from build123d import *

# Parameters (mm, degrees)
PIN_DRAWING_W       = 0.636
PIN_DRAWING_H       = 0.636
BOSS_EXTRUDE1_DEPTH = 2.54


with BuildPart() as part:
    # pin_drawing → Boss-Extrude1 (new body)
    with BuildSketch(Plane.XY):
        Polygon((0, 2.146446609), (0, 0.353553391), (0.353553391, 0), (0, -0.353553391), (0, -2.146446609), (0.353553391, -2.5), (2.187446609, -2.5), (2.541, -2.146446609), (2.541, -0.353553391), (2.187446609, 0), (2.541, 0.353553391), (2.541, 2.146446609), (2.187446609, 2.5), (2.541, 2.853553391), (2.541, 4.646446609), (2.187446609, 5), (2.541, 5.353553391), (2.541, 7.146446609), (2.187446609, 7.5), (0.353553391, 7.5), (0, 7.146446609), (0, 5.353553391), (0.353553391, 5), (0, 4.646446609), (0, 2.853553391), (0.353553391, 2.5), align=None)
        with Locations((1.2705, -1.25)):
            Rectangle(PIN_DRAWING_W, PIN_DRAWING_H, mode=Mode.SUBTRACT)
        with Locations((1.2705, 1.25)):
            Rectangle(PIN_DRAWING_W, PIN_DRAWING_H, mode=Mode.SUBTRACT)
        with Locations((1.2705, 3.75)):
            Rectangle(PIN_DRAWING_W, PIN_DRAWING_H, mode=Mode.SUBTRACT)
        with Locations((1.2705, 6.25)):
            Rectangle(PIN_DRAWING_W, PIN_DRAWING_H, mode=Mode.SUBTRACT)
    extrude(amount=BOSS_EXTRUDE1_DEPTH)


solid = part.part
Source: CAD feature listing. Evaluate the final solid. Frame: model axes, mm. Round coordinates to 2 decimals unless told otherwise and drop trailing zeros. Loops run counter-clockwise (first coordinate to the right, second up) from the corner with the lowest first, then second, coordinate; pieces in that order, holes last. Notation, with made-up numbers: M 64,10 L 118,10 A26 ccw 118,29 Z; hole C 75.25,44 d6. An arc over 180 degrees is marked long. Return JSON: item names as keys, results as strings. Group by question number.
1. Material intervals for line 1 along Y through (x, z) = (1, 1.5); line 2 along X through (y, z) = (1.25, 2.25); line 3 along Y through (x, z) = (0.2, 2.2), sorted ascending. Write a range as from..to.
2. Pin query (flat end, axial travel): pin 1 (0.7 mm diameter, centred on y = 3.5, z = 1, fed in from -X). Return the tip coordinate at first contact, or that it passes through.
3. Section query D-D on z = 1.2. State how many separate pieces and enclosed holes the cut face has, and give its area (3 significant figures).
4. Section query A-A on x = 1.05. Output: boundary loops of the cut face in (y, z).
5. Section query C-C on x = 2.35. Output: boundary loops of the cut face in (y, z).
6. Section query B-B on y = 3.75. Output: boundary loops of the cut face in (x, z).
Checks:
{
 "1": {"line 1": "y = -2.5..-1.57, -0.93..0.93, 1.57..3.43, 4.07..5.93, 6.57..7.5", "line 2": "x = 0..0.95, 1.59..2.54", "line 3": "y = -2.35..-0.15, 0.15..2.35, 2.65..4.85, 5.15..7.35"},
 "2": {"pin 1": "stops at x = 0"},
 "3": {"separate pieces": "1", "enclosed holes": "4", "area": "22.8 mm²"},
 "4": {"outline": "M -2.5,0 L -1.57,0 L -1.57,2.54 L -2.5,2.54 Z; M -0.93,0 L 0.93,0 L 0.93,2.54 L -0.93,2.54 Z; M 1.57,0 L 3.43,0 L 3.43,2.54 L 1.57,2.54 Z; M 4.07,0 L 5.93,0 L 5.93,2.54 L 4.07,2.54 Z; M 6.57,0 L 7.5,0 L 7.5,2.54 L 6.57,2.54 Z"},
 "5": {"outline": "M -2.34,0 L -0.16,0 L -0.16,2.54 L -2.34,2.54 Z; M 0.16,0 L 2.34,0 L 2.34,2.54 L 0.16,2.54 Z; M 2.66,0 L 4.84,0 L 4.84,2.54 L 2.66,2.54 Z; M 5.16,0 L 7.34,0 L 7.34,2.54 L 5.16,2.54 Z"},
 "6": {"outline": "M 0,0 L 0.95,0 L 0.95,2.54 L 0,2.54 Z; M 1.59,0 L 2.54,0 L 2.54,2.54 L 1.59,2.54 Z"}
}
